Read the model definition and answer for the solid it produces. Units are mm, in the model's axes. Give positions to 0.01 mm unless a question says otherwise; leave off trailing zeros. Loops run counter-clockwise (first coordinate to the right, second up) from the corner with the lowest first, then second, coordinate; pieces in that order, holes last. Notation, with made-up numbers: M 72.25,34.25 L 104.25,34.25 A22 cw 104.25,65.25 Z; hole C 22,-8 d4. An arc over 180 degrees is marked long. Return JSON: item names as keys, results as strings. Group by question number.
```python
from build123d import *

# Parameters (mm, degrees)
F1_DEPTH = 1
F2_SIZE  = 0.2
F3_SIZE  = 0.6


with BuildPart() as f1:
    # F0 (on Top) → F1 (new body)
    with BuildSketch(Plane.XY):
        with BuildLine():
            ThreePointArc((5, 1.6007810594), (5.1871234803, 0.8100925873), (5.25, 0))
            ThreePointArc((5.25, 0), (-0.8100925873, -5.1871234803), (-5, 1.6007810594))
            Line((-5, 1.6007810594), (-5, 9.7979589711))
            ThreePointArc((-5, 9.7979589711), (-5.7445626465, -9.3808315196), (11, 0))
            ThreePointArc((11, 0), (9.3808315196, 5.7445626465), (5, 9.7979589711))
            Line((5, 9.7979589711), (5, 1.6007810594))
        make_face()
    extrude(amount=F1_DEPTH)

    # F2
    f2_edges = [f1.edges().sort_by_distance(p)[0] for p in [
        (0, -5.25, 0),
        (-5, 5.69937, 0),
        (-5.744563, -9.380832, 0),
        (9.380832, 5.744563, 0),
        (5, 5.69937, 0),
    ]]
    chamfer(f2_edges, length=F2_SIZE)

    # F3
    f3_edges = [f1.edges().sort_by_distance(p)[0] for p in [
        (0, -5.25, 1),
        (-5, 5.69937, 1),
        (-5.744563, -9.380832, 1),
        (9.380832, 5.744563, 1),
        (5, 5.69937, 1),
    ]]
    chamfer(f3_edges, length=F3_SIZE)


solid = f1.part
```
1. Straight lines are drawn through the part: line 1 along X through (y, z) = (0, 0.3); line 2 along Y through (x, z) = (0, 0.3); line 3 along X through (y, z) = (-3, 0.15). For each, find the intervals that lie inside material, in ascending order.
2. A flat-ended cylindrical pin translates along its axis: P1, Ø8.5, axis at x = 0, y = 0, coming from the -Z side (3 decimals). Find the tip coordinate at first contact, or state that the pin passes through.
3. Find section A-A (x = 0). Write down the section's boundary in (y, z), and give its area (3 significant figures).
Result:
{
 "1": {"line 1": "x = -11 to -5.25, 5.25 to 11", "line 2": "y = -11 to -5.25", "line 3": "x = -10.53 to -4.37, 4.37 to 10.53"},
 "2": {"P1": "passes through"},
 "3": {"outline": "M -11,0.2 L -10.8,0 L -5.45,0 L -5.25,0.2 L -5.25,0.4 L -5.85,1 L -10.4,1 L -11,0.4 Z", "area": "5.35 mm2"}
}
